Source: CAD feature listing. Evaluate the final solid. Frame: model axes, mm. Face numbers are marked on the shaded views. A direction names the side the tool comes from. Give positions to 0.01 mm unless a question says otherwise; leave off trailing zeros. Order: outer loops, then holes, each group sorted by start corner. A loop starts at its lowest first (then second) coordinate and runs counter-clockwise, first axis right, second up.
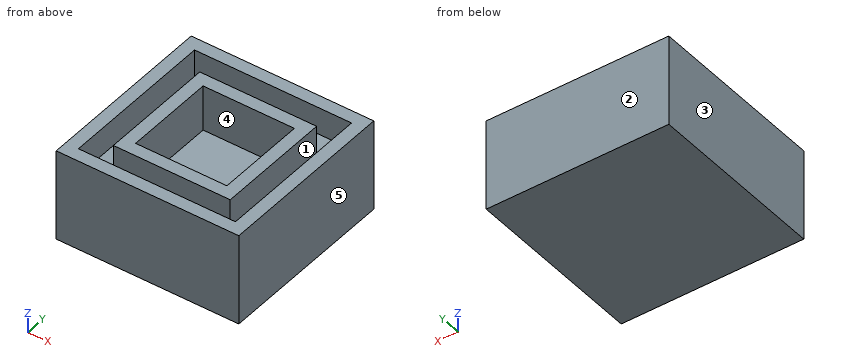
```python
from build123d import *

# Parameters (mm, degrees)
SKETCH_1_W          = 20
SKETCH_1_H          = 20
EXTRUDE_1_DEPTH     = 10
SHELL_1_T           = -5
SKETCH_3_W          = 17.2
SKETCH_3_H          = 17.2
SKETCH_3_W_2        = 12.8
SKETCH_3_H_2        = 12.8
CUT_EXTRUDE_1_DEPTH = 3


with BuildPart() as part:
    # ｽｹｯﾁ1 → ﾎﾞｽ - 押し出し1 (new body)
    with BuildSketch(Plane.XY):
        Rectangle(SKETCH_1_W, SKETCH_1_H)
    extrude(amount=EXTRUDE_1_DEPTH)

    # ｼｪﾙ1
    shell_1_openings = [part.faces().sort_by_distance(p)[0] for p in [
        (0, 0, 10),
    ]]
    offset(amount=SHELL_1_T, openings=shell_1_openings, kind=Kind.INTERSECTION)

    # ｽｹｯﾁ3 → ｶｯﾄ - 押し出し1 (cut)
    with BuildSketch(Plane.XY.offset(10)):
        Rectangle(SKETCH_3_W, SKETCH_3_H)
        Rectangle(SKETCH_3_W_2, SKETCH_3_H_2, mode=Mode.SUBTRACT)
    extrude(amount=-CUT_EXTRUDE_1_DEPTH, mode=Mode.SUBTRACT)


solid = part.part
```
1) Section query C-C, the plane y = -5.25. Return the cut outline in (x, z).
Report:
outline: (-10, 0) - (10, 0) - (10, 10) - (8.6, 10) - (8.6, 7) - (6.4, 7) - (6.4, 10) - (-6.4, 10) - (-6.4, 7) - (-8.6, 7) - (-8.6, 10) - (-10, 10) - close
2) Section query B-B, the plane x = -4. Return the cut outline in (y, z), and give its area (3 significant figures).
Report:
outline: (-10, 0) - (10, 0) - (10, 10) - (8.6, 10) - (8.6, 7) - (6.4, 7) - (6.4, 10) - (5, 10) - (5, 5) - (-5, 5) - (-5, 10) - (-6.4, 10) - (-6.4, 7) - (-8.6, 7) - (-8.6, 10) - (-10, 10) - close
area: 137 mm2
3) Section query A-A, the plane z = 9. Return the cut outline in (x, y).
Report:
outline: (-10, -10) - (10, -10) - (10, 10) - (-10, 10) - close; (-6.4, -6.4) - (6.4, -6.4) - (6.4, 6.4) - (-6.4, 6.4) - close; hole (-8.6, -8.6) - (8.6, -8.6) - (8.6, 8.6) - (-8.6, 8.6) - close; hole (-5, -5) - (5, -5) - (5, 5) - (-5, 5) - close
4) Pin query (flat end, axial travel): pin 1 (5 mm diameter, centred on x = -7, y = -7.5, fed in from +Z). Return the tip coordinate at first contact, or that it passes through.
Report:
pin 1: stops at z = 10
5) Draft query along Y for the marked faces 1, 2 and 3. Return one class per face: +Y half, -Y half, draft (parallel to the pull), parting line (faces both ways), or undercut.
Report:
face 1: undercut
face 2: +Y half
face 3: draft
6) Section query D-D, the plane z = 6. Return the cut outline in (x, y).
Report:
outline: (-10, -10) - (10, -10) - (10, 10) - (-10, 10) - close; hole (-5, -5) - (5, -5) - (5, 5) - (-5, 5) - close
7) Reachability of the marked faces 4 and 5 from +Z, -Z, +X, -X, +Y, -Y: full face, straight path, thin tool, end or side. Return the list, or none.
Report:
face 4: +Z
face 5: +Z, -Z, +X, +Y, -Y
8) Material intervals for L1, parallel to Y at x = 6, z = 8.75; L2, parallel to X at y = -1, z = 9.5; L3, parallel to X at y = -7.5, z = 8.75, sorted ascending.
Report:
L1: y = -10 to -8.6, -6.4 to 6.4, 8.6 to 10
L2: x = -10 to -8.6, -6.4 to -5, 5 to 6.4, 8.6 to 10
L3: x = -10 to -8.6, 8.6 to 10
